The model under review builds one solid part; all positions refer to its coordinate system, in mm. A direction names the side the tool comes from. Round coordinates to 2 decimals unless told otherwise and drop trailing zeros. Write each loop counter-clockwise with the first axis right and the second up, starting at its lowest first coordinate (ties: lowest second). Pieces come first, ordered by that corner, then holes. Notation, with made-up numbers: (56.25, 54) -> (108.25, 54) arc R26 cw to (108.25, 75) -> close; hole circle Ø10 at (9.25, 29). An arc over 180 degrees is marked (long way). Answer as a JSON object with one key per item and string values. Group by question number.
1) Machinability: for faces 4 (the cylindrical face through (1.29, 14.38, -2.024)), 5 (the cylindrical face through (2.003, 6.986, -0.631)), 6 (the cylindrical face through (-3, 3, 0)), which of the approach directions +Z, -Z, +X, -X, +Y, -Y give a long, thin tool a straight path to every point of the face, cutting with its end or side? Answer none if there is none.
2) Mouldability with a two-part tool opening along Y and no side actions: class faces 1 (the flat face through (1.3, 8, 2)), 2 (the cylindrical face through (-3, 10, 0)), 3 (the flat face through (0, 0, 2)) as pulls with the +Y half, pulls with the -Y half, needs draft (parallel to the pull), parting line crosses it, or undercut.
3) We need section A-A, the plane x = 0. Write out the cut boundary in (y, z).
4) To check wall thickness, follow probe 1 along X at (y, z) = (14.7, 0); probe 2 along Y at (x, z) = (0.2, -2.15); probe 3 along X at (y, z) = (3.5, 0). State the ranges of each line that lie inside material, in increasing order. Write a range as [from, to].
5) We need section C-C, the plane y = 7.25. Write out the cut boundary in (x, z), then the cut area to 3 significant figures.
6) We need section B-B, the plane z = 0. Write out the cut boundary in (x, y).
7) Insertion check: pin 1 Ø1.5 at (y, z) = (14, 0.5) entering from -X; pin 2 Ø1.8 at (x, z) = (1, -0.5) entering from -Y; pin 3 Ø1 at (x, y) = (0.5, 14) entering from +Z; pin 4 Ø1.5 at (y, z) = (4.5, 1.5) entering from +X. Each pin has a flat end and moves straight along its axis. Give the tip position at first contact, or say it passes through.
from build123d import *

# Parameters (mm, degrees)
SKETCH1_R               = 3
BOSS_EXTRUDE1_DEPTH     = 6
SKETCH2_R               = 2.1
BOSS_EXTRUDE2_DEPTH     = 2
SKETCH3_R               = 3
BOSS_EXTRUDE3_DEPTH     = 5
SKETCH4_R               = 1.6
CUT_EXTRUDE1_DEPTH      = 14
CROQUIS1_R              = 2.4
CROQUIS1_R_2            = 1.6
SALIENTE_EXTRUIR1_DEPTH = 3
CHAFL_N1_SIZE           = 0.2
CHAFL_N2_SIZE           = 0.2
CHAFL_N3_SIZE           = 0.25
CHAFL_N3_SIZE2          = 0.433012702


with BuildPart() as part:
    # Sketch1 → Boss-Extrude1 (new body)
    with BuildSketch(Plane(origin=(0, 0, 0), x_dir=(1, 0, 0), z_dir=(0, 1, 0))):
        Circle(SKETCH1_R)
    extrude(amount=BOSS_EXTRUDE1_DEPTH)

    # Sketch2 → Boss-Extrude2 (add)
    with BuildSketch(Plane(origin=(0, 6, 0), x_dir=(1, 0, 0), z_dir=(0, 1, 0))):
        Circle(SKETCH2_R)
    extrude(amount=BOSS_EXTRUDE2_DEPTH)

    # Sketch3 → Boss-Extrude3 (add)
    with BuildSketch(Plane(origin=(0, 8, 0), x_dir=(1, 0, 0), z_dir=(0, 1, 0))):
        Circle(SKETCH3_R)
    extrude(amount=BOSS_EXTRUDE3_DEPTH)

    # Sketch4 → Cut-Extrude1 (cut, through all)
    with BuildSketch(Plane(origin=(0, 13, 0), x_dir=(1, 0, 0), z_dir=(0, 1, 0))):
        Circle(SKETCH4_R)
    extrude(amount=-CUT_EXTRUDE1_DEPTH, mode=Mode.SUBTRACT)

    # Croquis1 → Saliente-Extruir1 (add)
    with BuildSketch(Plane(origin=(0, 13, 0), x_dir=(1, 0, 0), z_dir=(0, 1, 0))):
        Circle(CROQUIS1_R)
        Circle(CROQUIS1_R_2, mode=Mode.SUBTRACT)
    extrude(amount=SALIENTE_EXTRUIR1_DEPTH)

    # Chaflán1
    chafl_n1_edges = [part.edges().sort_by_distance(p)[0] for p in [
        (-2.4, 16, 0),
    ]]
    chamfer(chafl_n1_edges, length=CHAFL_N1_SIZE)

    # Chaflán2
    chafl_n2_edges = [part.edges().sort_by_distance(p)[0] for p in [
        (-3, 0, 0),
    ]]
    chamfer(chafl_n2_edges, length=CHAFL_N2_SIZE)

    # Chaflán3
    chafl_n3_edges = [part.edges().sort_by_distance(p)[0] for p in [
        (-1.6, 16, 0),
    ]]
    chafl_n3_side = [part.faces().sort_by_distance(p)[0] for p in [
        (-2.137774603, 16, 0),
    ]]
    chamfer(chafl_n3_edges, length=CHAFL_N3_SIZE, length2=CHAFL_N3_SIZE2, reference=chafl_n3_side[0])


solid = part.part
Here are the results:
{
 "1": {"face 4": "+Y", "face 5": "none", "face 6": "+Y, -Y"},
 "2": {"face 1": "undercut", "face 2": "needs draft", "face 3": "pulls with the -Y half"},
 "3": {"outline": "(0, -2.8) -> (0.2, -3) -> (6, -3) -> (6, -2.1) -> (8, -2.1) -> (8, -3) -> (13, -3) -> (13, -2.4) -> (15.8, -2.4) -> (16, -2.2) -> (16, -1.85) -> (15.57, -1.6) -> (0, -1.6) -> close; (0, 1.6) -> (15.57, 1.6) -> (16, 1.85) -> (16, 2.2) -> (15.8, 2.4) -> (13, 2.4) -> (13, 3) -> (8, 3) -> (8, 2.1) -> (6, 2.1) -> (6, 3) -> (0.2, 3) -> (0, 2.8) -> close"},
 "4": {"probe 1": "x = [-2.4, -1.6], [1.6, 2.4]", "probe 2": "y = [0, 6], [8, 16]", "probe 3": "x = [-3, -1.6], [1.6, 3]"},
 "5": {"outline": "circle Ø4.2 at (0, 0); hole circle Ø3.2 at (0, 0)", "area": "5.81 mm^2"},
 "6": {"outline": "(-3, 0.2) -> (-2.8, 0) -> (-1.6, 0) -> (-1.6, 15.57) -> (-1.85, 16) -> (-2.2, 16) -> (-2.4, 15.8) -> (-2.4, 13) -> (-3, 13) -> (-3, 8) -> (-2.1, 8) -> (-2.1, 6) -> (-3, 6) -> close; (1.6, 0) -> (2.8, 0) -> (3, 0.2) -> (3, 6) -> (2.1, 6) -> (2.1, 8) -> (3, 8) -> (3, 13) -> (2.4, 13) -> (2.4, 15.8) -> (2.2, 16) -> (1.85, 16) -> (1.6, 15.57) -> close"},
 "7": {"pin 1": "stops at x = -2.4", "pin 2": "stops at y = 0", "pin 3": "stops at z = 2.4", "pin 4": "stops at x = 2.9"}
}
